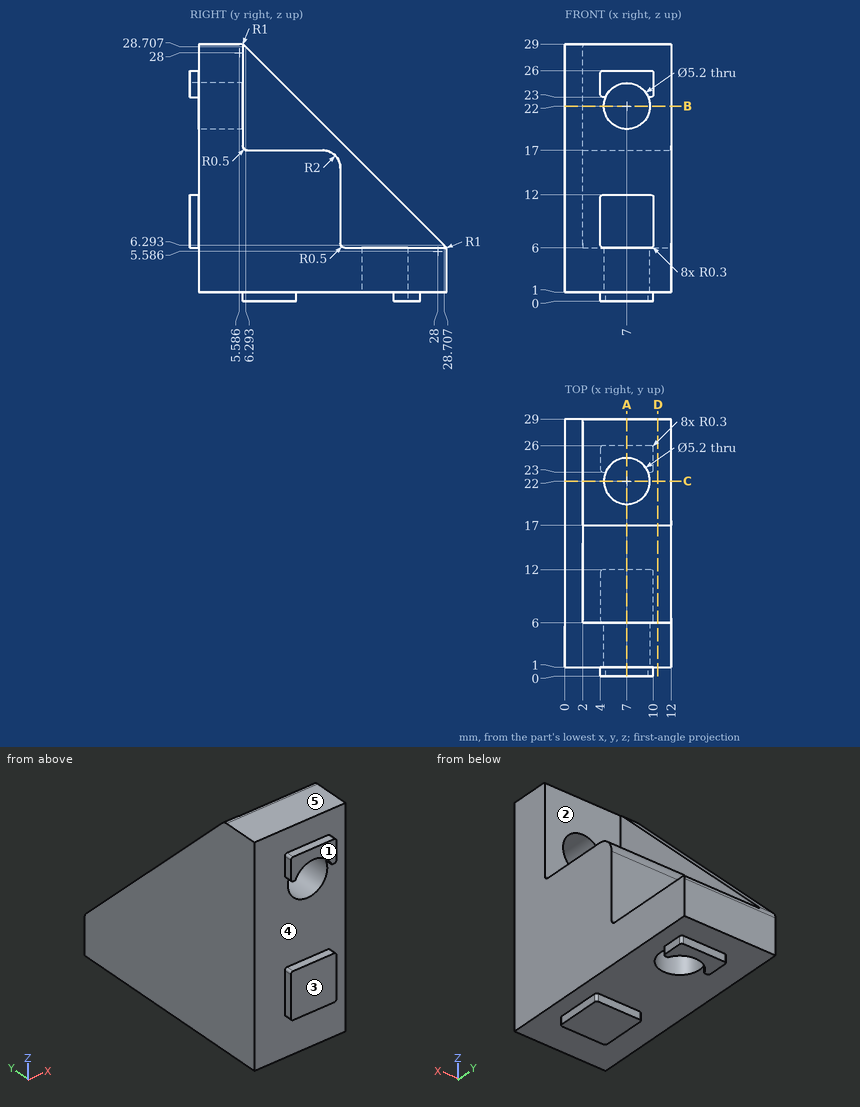
Geometry: see drawing. Coordinates: mm, zero at the bounding-box minimum. A direction names the side the tool comes from. Give positions to 0.01 mm unless a question says otherwise; leave off trailing zeros. Loops run counter-clockwise (first coordinate to the right, second up) from the corner with the lowest first, then second, coordinate; pieces in that order, holes last. Notation, with made-up numbers: M 77.25,-8 L 104.25,-8 A12 cw 104.25,2 Z; hole C 9,-38 d5. An arc over 180 degrees is marked long. Use one line per item in the form item = value.
1. Reachability of the marked faces 1 and 2 from +Z, -Z, +X, -X, +Y, -Y: full face, straight path, thin tool, end or side. Return the list, or none.
Numbers:
face_1 = +Z, -Z, +X, -X, -Y
face_2 = +Z, +X, +Y
2. Section query D-D, the plane x = 10.5. Return the cut outline in (y, z).
Numbers:
outline = M 1,1 L 29,1 L 29,5.59 A1 ccw 28.91,6 L 17.5,6 A0.5 cw 17,6.5 L 17,15 A2 ccw 15,17 L 6.5,17 A0.5 cw 6,17.5 L 6,28.91 A1 ccw 5.59,29 L 1,29 Z
3. First-contact query: pin 1 (4 mm diameter, centred on x = 6.5, z = 15.5, fed in from -Y); pin 2 (4 mm diameter, centred on x = 6.5, y = 9, fed in from +Z); pin 3 (1.5 mm diameter, centred on x = 3, z = 20, fed in from +Y). Flat tips, straight axial feed; report the tip coordinate or a pass-through.
Numbers:
pin_1 = 1
pin_2 = 17
pin_3 = 6
4. Line query: L1, parallel to X at y = 22, z = 1.45; L2, parallel to Z at x = 7, y = 3.1; L3, parallel to Y at x = 7.25, z = 25.25. Output: solid intervals per line, ascending.
Numbers:
L1 = 0 to 4.4, 9.6 to 12
L2 = 1 to 19.4, 24.6 to 29
L3 = 0 to 6
5. Section query B-B, the plane z = 22. Return the cut outline in (x, y), and give its area (3 significant figures).
Numbers:
outline = M 0,1 L 4.4,1 L 4.4,6 L 2,6 L 2,13 L 0,13 Z; M 9.6,1 L 12,1 L 12,6 L 9.6,6 Z
area = 48.0 mm²
6. Pull-direction query (Z, two-part tool) for the marked faces 3, 4 and 5; classes: released by +Z, released by -Z, zero draft, split by the parting line, or undercut.
Numbers:
face_3 = zero draft
face_4 = undercut
face_5 = released by +Z
7. Section query A-A, the plane x = 7. Count the separate pieces of the cut face and the enclosed holes in it, and give its area (3 significant figures).
Numbers:
separate_pieces = 3
enclosed_holes = 0
area = 338 mm²
